```python
from build123d import *

# Parameters (mm, degrees)
BOSS_EXTRUDE2_DEPTH         = 2
BOSS_EXTRUDE2_DEPTH_BACK    = 4
SKETCH2_W                   = 50
SKETCH2_H                   = 40
BOSS_EXTRUDE3_DEPTH         = 4
BOSS_EXTRUDE3_DEPTH_BACK    = 2
BOSS_EXTRUDE4_DEPTH         = 4
BOSS_EXTRUDE4_DEPTH_BACK    = 2
CUT_EXTRUDE1_DEPTH          = 10
CUT_EXTRUDE1_DEPTH_BACK     = 92
SKETCH7_R                   = 1.5
SKETCH7_R_2                 = 6
SKETCH8_R                   = 2.9
SKETCH8_R_2                 = 1.55
CUT_EXTRUDE2_DEPTH          = 92
SKETCH10_W                  = 4
SKETCH10_H                  = 6
BOSS_EXTRUDE5_DEPTH         = 40
IZIM1_R                     = 2.313202435
KES_EKSTR_ZYON1_DEPTH       = 48
Y_KSEKLIK_EKSTR_ZYON1_DEPTH = 6
IZIM3_R                     = 8
KES_EKSTR_ZYON2_DEPTH       = 6


with BuildPart() as part:
    # Sketch2 → Boss-Extrude2 (new, two sides: drawn at the far end of the back side and taken through both)
    with BuildSketch(Plane(origin=(0, 0, 0), x_dir=(1, 0, 0), z_dir=(0, 1, 0)).offset(-BOSS_EXTRUDE2_DEPTH_BACK)):
        with Locations((3.5, 41.570780176)):
            Rectangle(SKETCH2_W, SKETCH2_H)
    extrude(amount=BOSS_EXTRUDE2_DEPTH + BOSS_EXTRUDE2_DEPTH_BACK)

    # Sketch4 → Boss-Extrude3 (add, two sides: drawn at the far end of the back side and taken through both)
    with BuildSketch(Plane.ZY.offset(21.5).offset(-BOSS_EXTRUDE3_DEPTH_BACK)):
        with BuildLine():
            Line((-21.570780176, 2), (-61.570780176, 2))
            Line((-61.570780176, 2), (-61.570780176, 32))
            ThreePointArc((-61.570780176, 32), (-41.570780176, 52), (-21.570780176, 32))
            Line((-21.570780176, 32), (-21.570780176, 2))
        make_face()
    extrude(amount=BOSS_EXTRUDE3_DEPTH + BOSS_EXTRUDE3_DEPTH_BACK)

    # Sketch5 → Boss-Extrude4 (add, two sides: drawn at the far end of the back side and taken through both)
    with BuildSketch(Plane(origin=(28.5, 0, 0), x_dir=(0, 0, -1), z_dir=(1, 0, 0)).offset(-BOSS_EXTRUDE4_DEPTH_BACK)):
        with BuildLine():
            Line((21.570780176, -4), (61.570780176, -4))
            Line((61.570780176, -4), (61.570780176, 32))
            ThreePointArc((61.570780176, 32), (41.570780176, 52), (21.570780176, 32))
            Line((21.570780176, 32), (21.570780176, -4))
        make_face()
    extrude(amount=BOSS_EXTRUDE4_DEPTH + BOSS_EXTRUDE4_DEPTH_BACK)

    # Sketch7 → Cut-Extrude1 (cut, two sides: drawn at the far end of the back side and taken through both)
    with BuildSketch(Plane.ZY.offset(21.5).offset(-CUT_EXTRUDE1_DEPTH_BACK)):
        with Locations(Location((-26.070780176, 32, 0), (0, 0, 180))):
            Circle(SKETCH7_R)
        with Locations(Location((-33.820780176, 18.576606241, 0), (0, 0, 180))):
            Circle(SKETCH7_R)
        with Locations(Location((-49.320780176, 18.576606241, 0), (0, 0, 180))):
            Circle(SKETCH7_R)
        with Locations(Location((-57.070780176, 32, 0), (0, 0, 180))):
            Circle(SKETCH7_R)
        with Locations(Location((-49.320780176, 45.423393759, 0), (0, 0, 180))):
            Circle(SKETCH7_R)
        with Locations(Location((-33.820780176, 45.423393759, 0), (0, 0, 180))):
            Circle(SKETCH7_R)
        with Locations(Location((-41.570780176, 39, 0), (0, 0, 180))):
            Circle(SKETCH7_R_2)
    extrude(amount=CUT_EXTRUDE1_DEPTH + CUT_EXTRUDE1_DEPTH_BACK, mode=Mode.SUBTRACT)

    # Sketch8 → Cut-Extrude2 (cut)
    with BuildSketch(Plane(origin=(0, 2, 0), x_dir=(1, 0, 0), z_dir=(0, 1, 0))):
        with Locations(Location((3.5, 41.570780176, 0), (0, 0, 270))):
            Circle(SKETCH8_R)
        with Locations(Location((-1.49, 46.560780176, 0), (0, 0, 270))):
            Circle(SKETCH8_R_2)
        with Locations(Location((8.49, 46.560780176, 0), (0, 0, 270))):
            Circle(SKETCH8_R_2)
        with Locations(Location((-1.49, 36.580780176, 0), (0, 0, 270))):
            Circle(SKETCH8_R_2)
        with Locations(Location((8.49, 36.580780176, 0), (0, 0, 270))):
            Circle(SKETCH8_R_2)
    extrude(amount=-CUT_EXTRUDE2_DEPTH, mode=Mode.SUBTRACT)

    # Sketch10 → Boss-Extrude5 (add)
    with BuildSketch(Plane.XY.offset(-21.570780176)):
        with Locations((-23.5, -1)):
            Rectangle(SKETCH10_W, SKETCH10_H)
    extrude(amount=-BOSS_EXTRUDE5_DEPTH)

    # Çizim1 → Kes-Ekstrüzyon1 (cut)
    with BuildSketch(Plane(origin=(-19.5, 0, 0), x_dir=(0, 0, -1), z_dir=(1, 0, 0))):
        with Locations((26.070780176, 32)):
            Circle(IZIM1_R)
        with Locations((33.820780176, 45.423393759)):
            Circle(IZIM1_R)
        with Locations((49.320780176, 45.423393759)):
            Circle(IZIM1_R)
        with Locations((57.070780176, 32)):
            Circle(IZIM1_R)
        with Locations((49.320780176, 18.576606241)):
            Circle(IZIM1_R)
        with Locations((33.820780176, 18.576606241)):
            Circle(IZIM1_R)
    extrude(amount=KES_EKSTR_ZYON1_DEPTH, mode=Mode.SUBTRACT)

    # Çizim2 → Yükseklik-Ekstrüzyon1 (add)
    with BuildSketch(Plane.ZY.offset(25.5)):
        with BuildLine():
            Line((-21.570780176, -4), (-21.570780176, 32))
            ThreePointArc((-21.570780176, 32), (-41.570780176, 52), (-61.570780176, 32))
            Line((-61.570780176, 32), (-61.570780176, -4))
            Line((-61.570780176, -4), (-21.570780176, -4))
        make_face()
    extrude(amount=-Y_KSEKLIK_EKSTR_ZYON1_DEPTH)

    # Çizim3 → Kes-Ekstrüzyon2 (cut)
    with BuildSketch(Plane.ZY.offset(25.5)):
        with Locations((-41.570780176, 39)):
            Circle(IZIM3_R)
    extrude(amount=-KES_EKSTR_ZYON2_DEPTH, mode=Mode.SUBTRACT)


solid = part.part
```
Input: part model. Units: mm. Frame: model coordinates. A direction names the side the tool comes from. Coordinates: 2 decimals unless noted, no trailing zeros. Write each loop counter-clockwise with the first axis right and the second up, starting at its lowest first coordinate (ties: lowest second). Pieces come first, ordered by that corner, then holes. Notation, with made-up numbers: (26.25, 53) -> (79.25, 53) arc R21 cw to (79.25, 74) -> close; hole circle Ø2 at (1, 66). An arc over 180 degrees is marked (long way). Answer as a JSON object with one key per item and string values.
1. Section D-D on z = -43. Return the cut outline in (x, y), then the cut area to 3 significant figures.
Result set:
{"outline": "(-25.5, -4) -> (0.98, -4) -> (0.98, 2) -> (-19.5, 2) -> (-19.5, 31.13) -> (-25.5, 31.13) -> close; (-25.5, 46.87) -> (-19.5, 46.87) -> (-19.5, 51.95) -> (-25.5, 51.95) -> close; (6.02, -4) -> (32.5, -4) -> (32.5, 33.17) -> (26.5, 33.17) -> (26.5, 2) -> (6.02, 2) -> close; (26.5, 44.83) -> (32.5, 44.83) -> (32.5, 51.95) -> (26.5, 51.95) -> close", "area": "753 mm2"}
2. Section A-A on y = 14. Return the cut outline in (x, z), then the cut area to 3 significant figures.
Result set:
{"outline": "(-25.5, -61.57) -> (-19.5, -61.57) -> (-19.5, -21.57) -> (-25.5, -21.57) -> close; (26.5, -61.57) -> (32.5, -61.57) -> (32.5, -21.57) -> (26.5, -21.57) -> close", "area": "480 mm2"}
3. Access query for faces 1 (the face through (8, 1, -21.571)), 2 (the face through (30.528, 44.41, -32.715)), 3 (the face through (27.486, 20.14, -47.616)). Directions: +Z, -Z, +X, -X, +Y, -Y. A direction counts if a zero-diameter tool reaches every point of the face in a straight line with its end or side. Return the directions, or none.
Result set:
{"face 1": "+Z, +X, -X, +Y, -Y", "face 2": "+X", "face 3": "none"}
4. Mould query, pull axis Y, two halves, no side actions, for faces 4 (the face through (28.5, 17, -33)), 5 (the face through (-19.5, 22, -41)), 6 (the face through (29.458, 51.995, -42.011)). Classes: released by +Y, released by -Y, zero draft, split by the parting line, or undercut.
Result set:
{"face 4": "undercut", "face 5": "zero draft", "face 6": "released by +Y"}
5. Section B-B on x = 8.49. Return the cut outline in (y, z).
Result set:
{"outline": "(-4, -61.57) -> (2, -61.57) -> (2, -48.11) -> (-4, -48.11) -> close; (-4, -45.01) -> (2, -45.01) -> (2, -38.13) -> (-4, -38.13) -> close; (-4, -35.03) -> (2, -35.03) -> (2, -21.57) -> (-4, -21.57) -> close"}
6. First-contact query: P1, Ø3, axis at x = 1, z = -57, coming from the +Y side. Flat tip, straight axial feed; report the tip coordinate or a pass-through.
Result set:
{"P1": "stops at y = 2"}
7. Material intervals for line 1 (Z direction, x = 27, y = 32); line 2 (X direction, y = 10.5, z = -49); line 3 (Z direction, x = 8, y = 0), sorted ascending. Write a range as from..to.
Result set:
{"line 1": "z = -61.57..-59.38, -54.76..-28.38, -23.76..-21.57", "line 2": "x = -25.5..-19.5, 26.5..32.5", "line 3": "z = -61.57..-48.03, -45.09..-38.05, -35.11..-21.57"}
8. Section C-C on y = 0.5. Return the cut outline in (x, z).
Result set:
{"outline": "(-25.5, -61.57) -> (32.5, -61.57) -> (32.5, -21.57) -> (-25.5, -21.57) -> close; hole circle Ø3.1 at (-1.49, -46.56); hole circle Ø3.1 at (-1.49, -36.58); hole circle Ø5.8 at (3.5, -41.57); hole circle Ø3.1 at (8.49, -46.56); hole circle Ø3.1 at (8.49, -36.58)"}
